Autodesk Inventor part; units mm, degrees
ref_plane "Work Plane1" through (-10.187, -10.187, 3.6) normal (0, 0, -1) x (0.5228, 0.8525, 0)
ref_plane "YZ Plane" through (0, 0, 0) normal (1, 0, 0) x (0, 1, 0)
ref_plane "XZ Plane" through (0, 0, 0) normal (0, 1, 0) x (-1, 0, 0)
sketch "Sketch1" plane through (0, 0, 0) normal (0, 0, 1) x (1, 0, 0)
  circle A0 centre (0, 0) radius 1.525
  line L0 (3.3712, -2.153) -> (-0.0331, -3.9999)
  arc A1 (-0.1789, -3.996) -> (-0.0331, -3.9999) centre (0, 0) ccw
  line L1 (-0.1789, -3.996) -> (-3.4805, -1.9713)
  arc A2 (-3.5501, -1.843) -> (-3.4805, -1.9713) centre (0, 0) ccw
  line L2 (-3.5501, -1.843) -> (-3.4474, 2.0286)
  arc A3 (-3.3712, 2.153) -> (-3.4474, 2.0286) centre (0, 0) ccw
  line L3 (-3.3712, 2.153) -> (0.0331, 3.9999)
  arc A4 (0.1789, 3.996) -> (0.0331, 3.9999) centre (0, 0) ccw
  line L4 (0.1789, 3.996) -> (3.4805, 1.9713)
  arc A5 (3.5501, 1.843) -> (3.4805, 1.9713) centre (0, 0) ccw
  line L5 (3.5501, 1.843) -> (3.4474, -2.0286)
  arc A6 (3.3712, -2.153) -> (3.4474, -2.0286) centre (0, 0) ccw
  circle A7 centre (0, 0) radius 5
  point P0 (0, 0)
  dimension "d0" = 10
ref_plane "Work Plane1" through (-10.187, -10.187, 3.6) normal (0, 0, -1) x (0.5228, 0.8525, 0)
extrude "Extrusion1" add sketch "Sketch1" along normal up to surface (3.6 mm away) contours A7
properties part number "Servo_Spacer"
Build history of the part. All positions in model axes, mm. A direction names the side the tool comes from. Give positions to 0.01 mm unless a question says otherwise; leave off trailing zeros. Loops run counter-clockwise (first coordinate to the right, second up) from the corner with the lowest first, then second, coordinate; pieces in that order, holes last. Notation, with made-up numbers: (-7.5, -35) - (16.5, -35) arc R21 cw to (16.5, -30) - close; hole circle Ø7 at (31.25, 46.5). An arc over 180 degrees is marked (long way). Use a Markdown table: item, result.
(1) Which spindle directions (+Z, -Z, +X, -X, +Y, -Y) get a long thin tool onto all of the face, cutting with end or side? Do faces 4 (the face through (-1.8, -3, 1.8)), 5 (the face through (-3, -3, 3.6)). Say none if no direction does.
Taken from the geometry:
| item | result |
|---|---|
| face 4 | +Z, -Z |
| face 5 | +Z, +X, -X, +Y, -Y |
(2) Band-saw the part on B-B (z = 1.95). Give the cut face in (x, y).
Taken from the geometry:
| item | result |
|---|---|
| outline | circle Ø10 at (0, 0); hole (-3.55, -1.84) arc R4.02 ccw to (-3.48, -1.97) - (-0.18, -4) arc R4.11 ccw to (-0.03, -4) - (3.37, -2.15) arc R3.78 ccw to (3.45, -2.03) - (3.55, 1.84) arc R4.02 ccw to (3.48, 1.97) - (0.18, 4) arc R4.11 ccw to (0.03, 4) - (-3.37, 2.15) arc R3.78 ccw to (-3.45, 2.03) - close |
(3) Band-saw the part on A-A (y = -1.25). Give the cut face in (x, z).
Taken from the geometry:
| item | result |
|---|---|
| outline | (-4.84, 0) - (-3.53, 0) - (-3.53, 3.6) - (-4.84, 3.6) - close; (3.47, 0) - (4.84, 0) - (4.84, 3.6) - (3.47, 3.6) - close |
(4) Wall check: line 1 along Y through (x, z) = (-1, 3.15); line 2 along Y through (x, z) = (2.25, 1.1); line 3 along X through (y, z) = (3.5, 2.6). Give the ranges that are in metal, low to high.
Taken from the geometry:
| item | result |
|---|---|
| line 1 | -4.9 to -3.49, 3.44 to 4.9 |
| line 2 | -4.47 to -2.76, 2.73 to 4.47 |
| line 3 | -3.57 to -0.89, 0.99 to 3.57 |
(5) Drop a flat-ended pin along its axis: pin 1 Ø1.5 at (x, z) = (-2, 2) entering from -Y. Give the stop position or say it passes through.
Taken from the geometry:
| item | result |
|---|---|
| pin 1 | y = -4.84 |
(6) Band-saw the part on C-C (y = 0.75). Give the cut face in (x, z).
Taken from the geometry:
| item | result |
|---|---|
| outline | (-4.94, 0) - (-3.48, 0) - (-3.48, 3.6) - (-4.94, 3.6) - close; (3.52, 0) - (4.94, 0) - (4.94, 3.6) - (3.52, 3.6) - close |
(7) Pull direction X, two halves, no side cores. Call faces 1 (the face through (-3, -3, 0)), 2 (the face through (-1.693, 3.064, 1.775)), 3 (the face through (-1.08, 4.88, 1.77)): +X half, -X half, draft (parallel to the pull), parting line (faces both ways), or undercut.
Taken from the geometry:
| item | result |
|---|---|
| face 1 | draft |
| face 2 | undercut |
| face 3 | parting line |
